Input: part model. Units: mm. Frame: model coordinates. Coordinates: 2 decimals unless noted, no trailing zeros. Order: outer loops, then holes, each group sorted by start corner. A loop starts at its lowest first (then second) coordinate and runs counter-clockwise, first axis right, second up.
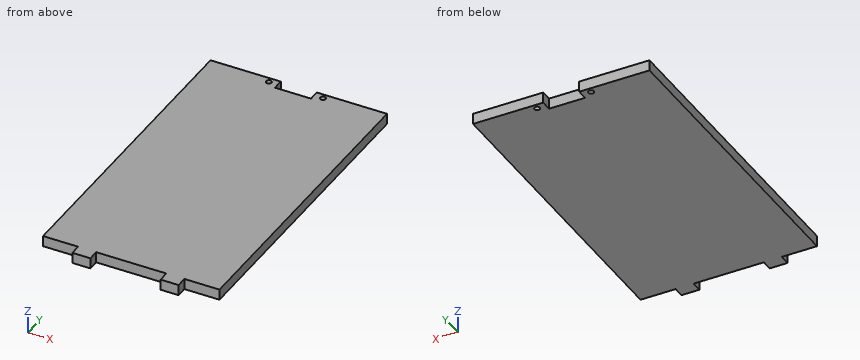
from build123d import *

# Parameters (mm, degrees)
ESQUISSE1_W             = 98
ESQUISSE1_H             = 173
BOSS_EXTRU_1_DEPTH      = 6
ESQUISSE2_W             = 10
ESQUISSE2_H             = 6
BOSS_EXTRU_2_DEPTH      = 6
ESQUISSE3_R             = 1.5
ENL_V_MAT_EXTRU_1_DEPTH = 6
ESQUISSE4_W             = 20
ESQUISSE4_H             = 6
ENL_V_MAT_EXTRU_2_DEPTH = 6


with BuildPart() as part:
    # Esquisse1 → Boss.-Extru.1 (new body)
    with BuildSketch(Plane.XY):
        Rectangle(ESQUISSE1_W, ESQUISSE1_H)
    extrude(amount=BOSS_EXTRU_1_DEPTH)

    # Esquisse2 → Boss.-Extru.2 (add)
    with BuildSketch(Plane.XY.offset(6)):
        with Locations((24.5, -89.5)):
            Rectangle(ESQUISSE2_W, ESQUISSE2_H)
        with Locations((-24.5, -89.5)):
            Rectangle(ESQUISSE2_W, ESQUISSE2_H)
    extrude(amount=-BOSS_EXTRU_2_DEPTH)

    # Esquisse3 → Enlèv. mat.-Extru.1 (cut)
    with BuildSketch(Plane.XY.offset(6)):
        with Locations((-15, 83.5)):
            Circle(ESQUISSE3_R)
        with Locations((15, 83.5)):
            Circle(ESQUISSE3_R)
    extrude(amount=-ENL_V_MAT_EXTRU_1_DEPTH, mode=Mode.SUBTRACT)

    # Esquisse4 → Enlèv. mat.-Extru.2 (cut)
    with BuildSketch(Plane.XY.offset(6)):
        with Locations((0, 83.5)):
            Rectangle(ESQUISSE4_W, ESQUISSE4_H)
    extrude(amount=-ENL_V_MAT_EXTRU_2_DEPTH, mode=Mode.SUBTRACT)


solid = part.part
Item 1: Cut plane C-C on x = -8. Return loops of the section in (y, z).
Response values:
outline: (-86.5, 0) - (80.5, 0) - (80.5, 6) - (-86.5, 6) - close
Item 2: Cut plane B-B on x = -33.5. Return loops of the section in (y, z).
Response values:
outline: (-86.5, 0) - (86.5, 0) - (86.5, 6) - (-86.5, 6) - close
Item 3: Ray query, probe 1 along X at (y, z) = (83.5, 1.6); probe 2 along Y at (x, z) = (-15, 2.5); probe 3 along Y at (x, z) = (-11.5, 4.55). Return the intervals inside material, ascending.
Response values:
probe 1: x = -49 to -16.5, -13.5 to -10, 10 to 13.5, 16.5 to 49
probe 2: y = -86.5 to 82, 85 to 86.5
probe 3: y = -86.5 to 86.5
Item 4: Pin query (flat end, axial travel): pin 1 Ø6 at (x, y) = (8, -23.5) entering from -Z; pin 2 Ø2 at (x, z) = (10, 4.5) entering from -Y; pin 3 Ø1.8 at (y, z) = (-89, 2) entering from -X; pin 4 Ø1.8 at (x, y) = (-15, 83.5) entering from +Z. Return the tip coordinate at first contact, or that it passes through.
Response values:
pin 1: stops at z = 0
pin 2: stops at y = -86.5
pin 3: stops at x = -29.5
pin 4: passes through
Item 5: Cut plane A-A on z = 1.9. Return loops of the section in (x, y).
Response values:
outline: (-49, -86.5) - (-29.5, -86.5) - (-29.5, -92.5) - (-19.5, -92.5) - (-19.5, -86.5) - (19.5, -86.5) - (19.5, -92.5) - (29.5, -92.5) - (29.5, -86.5) - (49, -86.5) - (49, 86.5) - (10, 86.5) - (10, 80.5) - (-10, 80.5) - (-10, 86.5) - (-49, 86.5) - close; hole circle Ø3 at (-15, 83.5); hole circle Ø3 at (15, 83.5)
